from build123d import *

# Parameters (mm, degrees)
SKETCH_1_W          = 6
SKETCH_1_H          = 50
SKETCH_2_W          = 10
SKETCH_2_H          = 3
SKETCH_3_R          = 1
CUT_EXTRUDE_1_DEPTH = 5000


with BuildPart() as part:
    # 草图1 → 旋转1 (revolve)
    with BuildSketch(Plane.XY, mode=Mode.PRIVATE) as revolve_1_sk:
        with Locations((3, 0)):
            Rectangle(SKETCH_1_W, SKETCH_1_H)
    revolve(revolve_1_sk.sketch.rotate(Axis((0, 25, 0), (0, -1, 0)), 180), axis=Axis((0, 25, 0), (0, -1, 0)))

    # 草图2 → 旋转2 (revolve)
    with BuildSketch(Plane.XY):
        with Locations((5, 26.5)):
            Rectangle(SKETCH_2_W, SKETCH_2_H)
        with Locations((5, -26.5)):
            Rectangle(SKETCH_2_W, SKETCH_2_H)
    revolve(axis=Axis((0, 25, 0), (0, 1, 0)))

    # 草图3 → 切除-拉伸1 (cut)
    with BuildSketch(Plane(origin=(0, 28, 0), x_dir=(1, 0, 0), z_dir=(0, 1, 0))):
        with Locations(Location((-5, 5, 0), (0, 0, 180))):
            Circle(SKETCH_3_R)
        with Locations(Location((5, 5, 0), (0, 0, 180))):
            Circle(SKETCH_3_R)
        with Locations(Location((-5, -5, 0), (0, 0, 180))):
            Circle(SKETCH_3_R)
        with Locations(Location((5, -5, 0), (0, 0, 180))):
            Circle(SKETCH_3_R)
    extrude(amount=-CUT_EXTRUDE_1_DEPTH, mode=Mode.SUBTRACT)


solid = part.part
Build history of the part. All positions in model axes, mm. A direction names the side the tool comes from. Coordinates: 2 decimals unless noted, no trailing zeros. Order: outer loops, then holes, each group sorted by start corner. A loop starts at its lowest first (then second) coordinate and runs counter-clockwise, first axis right, second up. Notation, with made-up numbers: (43, -6.75) - (92, -6.75) arc R13 ccw to (92, 15.25) - close; hole circle Ø7 at (54, 12). An arc over 180 degrees is marked (long way). Write item = value, one per line. Start each with the question number.
1) Saw through at C-C on x = 0. Write the cut outline in (y, z).
2) Saw through at B-B on z = -8.25. Write the cut outline in (x, y), then the cut area to 3 significant figures.
3) Saw through at D-D on z = -5. Write the cut outline in (x, y), then the cut area to 3 significant figures.
4) Flat gauge pins, fed straight in: pin 1 Ø1.6 at (x, z) = (-5, 5) entering from -Y; pin 2 Ø2.5 at (x, z) = (-5, -5) entering from -Y; pin 3 Ø3 at (y, z) = (-16.5, 1.5) entering from -X; pin 4 Ø6 at (y, z) = (-8.5, 5) entering from -X. Where does each tip first touch, or does it go through?
5) Two-plate mould, pull along Z, no slides. Class faces 3 (the face through (5, 27, -4)), 4 (the face through (-5, 27, -4)), 5 (the face through (-2.17, 26.52, 9.76)), 6 (the face through (0, 28, 0)): pulls with the +Z half, pulls with the -Z half, needs draft (parallel to the pull), parting line crosses it, or undercut.
6) Wall check: line 1 along Y through (x, z) = (-2.5, 7.75); line 2 along Z through (x, y) = (-5, 27.3); line 3 along Z through (x, y) = (2, -9). Give the ranges that are in metal, low to high. Write a range as from..to.
7) 3-axis set-ups, long thin cutter, end or side, ignore diameter. For faces 1 (the face through (-7, -25, 0)), 2 (the face through (-2.17, -26.48, 9.76)): which of +Z, -Z, +X, -X, +Y, -Y reach the whole face in a straight line?
8) Saw through at A-A on x = 8. Write the cut outline in (y, z), then the cut area to 3 significant figures.
From the geometry:
q1.outline = (-28, -10) - (-25, -10) - (-25, -6) - (25, -6) - (25, -10) - (28, -10) - (28, 10) - (25, 10) - (25, 6) - (-25, 6) - (-25, 10) - (-28, 10) - close
q2.outline = (-5.65, -28) - (5.65, -28) - (5.65, -25) - (-5.65, -25) - close; (-5.65, 25) - (5.65, 25) - (5.65, 28) - (-5.65, 28) - close
q2.area = 67.8 mm^2
q3.outline = (-8.66, -28) - (-6, -28) - (-6, -25) - (-8.66, -25) - close; (-8.66, 25) - (-6, 25) - (-6, 28) - (-8.66, 28) - close; (-4, -28) - (4, -28) - (4, -25) - (3.32, -25) - (3.32, 25) - (4, 25) - (4, 28) - (-4, 28) - (-4, 25) - (-3.32, 25) - (-3.32, -25) - (-4, -25) - close; (6, -28) - (8.66, -28) - (8.66, -25) - (6, -25) - close; (6, 25) - (8.66, 25) - (8.66, 28) - (6, 28) - close
q3.area = 412 mm^2
q4.pin_1 = through
q4.pin_2 = -28
q4.pin_3 = -6
q4.pin_4 = -5.66
q5.face_3 = undercut
q5.face_4 = undercut
q5.face_5 = parting line crosses it
q5.face_6 = needs draft
q6.line_1 = -28..-25, 25..28
q6.line_2 = -8.66..-6, -4..4, 6..8.66
q6.line_3 = -5.66..5.66
q7.face_1 = none
q7.face_2 = +Y, -Y
q8.outline = (-28, -6) - (-25, -6) - (-25, 6) - (-28, 6) - close; (25, -6) - (28, -6) - (28, 6) - (25, 6) - close
q8.area = 72.0 mm^2
